Here's how the part is built. I have some questions about the finished solid (model axes, mm). A direction names the side the tool comes from. Round coordinates to 2 decimals unless told otherwise and drop trailing zeros. Loops run counter-clockwise (first coordinate to the right, second up) from the corner with the lowest first, then second, coordinate; pieces in that order, holes last. Notation, with made-up numbers: M -38.75,-12 L 17.25,-12 A25 cw 17.25,9 Z; hole C 65.5,-34 d5. An arc over 180 degrees is marked long. Use a Markdown table: item, result.
from build123d import *

# Parameters (mm, degrees)
SKETCH1_R           = 2.6605
SKETCH1_R_2         = 2.41215
BOSS_EXTRUDE1_DEPTH = 4.5
BOSS_EXTRUDE2_DEPTH = 22.5
SKETCH3_R           = 2.6605
SKETCH3_R_2         = 4.25
BOSS_EXTRUDE3_DEPTH = 4
CUT_EXTRUDE2_DEPTH  = 59.403767002
FILLET1_R           = 4


with BuildPart() as part:
    # Sketch1 → Boss-Extrude1 (new body)
    with BuildSketch(Plane(origin=(0, 0, 0), x_dir=(1, 0, 0), z_dir=(0, 1, 0))):
        with BuildLine():
            Line((-31, -35), (31, -35))
            ThreePointArc((31, -35), (33.828427125, -33.828427125), (35, -31))
            Line((35, -31), (35, 31))
            ThreePointArc((35, 31), (33.828427125, 33.828427125), (31, 35))
            Line((31, 35), (-31, 35))
            ThreePointArc((-31, 35), (-33.828427125, 33.828427125), (-35, 31))
            Line((-35, 31), (-35, -31))
            ThreePointArc((-35, -31), (-33.828427125, -33.828427125), (-31, -35))
        make_face()
        with Locations(Location((25, 22.5, 0), (0, 0, 270))):
            Circle(SKETCH1_R, mode=Mode.SUBTRACT)
        with Locations(Location((25, -22.5, 0), (0, 0, 270))):
            Circle(SKETCH1_R, mode=Mode.SUBTRACT)
        with Locations(Location((-15, -22.5, 0), (0, 0, 270))):
            Circle(SKETCH1_R, mode=Mode.SUBTRACT)
        with Locations(Location((-15, 22.5, 0), (0, 0, 270))):
            Circle(SKETCH1_R, mode=Mode.SUBTRACT)
        with Locations(Location((-12, 0, 0), (0, 0, 270))):
            Circle(SKETCH1_R_2, mode=Mode.SUBTRACT)
        with Locations(Location((-27, 0, 0), (0, 0, 270))):
            Circle(SKETCH1_R_2, mode=Mode.SUBTRACT)
    extrude(amount=BOSS_EXTRUDE1_DEPTH)

    # Sketch2 → Boss-Extrude2 (add)
    with BuildSketch(Plane(origin=(0, 4.5, 0), x_dir=(1, 0, 0), z_dir=(0, 1, 0))):
        with BuildLine():
            Line((-27.289833197, 35), (-31, 35))
            ThreePointArc((-31, 35), (-33.828427125, 33.828427125), (-35, 31))
            Line((-35, 31), (-35, 17))
            Line((-35, 17), (-31.1, 17))
            Line((-31.1, 17), (-31.1, 31))
            ThreePointArc((-31.1, 31), (-31.070710678, 31.070710678), (-31, 31.1))
            Line((-31, 31.1), (-27.289833197, 31.1))
            Line((-27.289833197, 31.1), (-27.289833197, 35))
        make_face()
        with BuildLine():
            Line((-31, -35), (-27.289833197, -35))
            Line((-27.289833197, -35), (-27.289833197, -31.1))
            Line((-27.289833197, -31.1), (-31, -31.1))
            ThreePointArc((-31, -31.1), (-31.070710678, -31.070710678), (-31.1, -31))
            Line((-31.1, -31), (-31.1, -17))
            Line((-31.1, -17), (-35, -17))
            Line((-35, -17), (-35, -31))
            ThreePointArc((-35, -31), (-33.828427125, -33.828427125), (-31, -35))
        make_face()
        with BuildLine():
            Line((17, -35), (31, -35))
            ThreePointArc((31, -35), (33.828427125, -33.828427125), (35, -31))
            Line((35, -31), (35, 31))
            ThreePointArc((35, 31), (33.828427125, 33.828427125), (31, 35))
            Line((31, 35), (17, 35))
            Line((17, 35), (17, 31.1))
            Line((17, 31.1), (31, 31.1))
            ThreePointArc((31, 31.1), (31.070710678, 31.070710678), (31.1, 31))
            Line((31.1, 31), (31.1, -31))
            ThreePointArc((31.1, -31), (31.070710678, -31.070710678), (31, -31.1))
            Line((31, -31.1), (17, -31.1))
            Line((17, -31.1), (17, -35))
        make_face()
    extrude(amount=BOSS_EXTRUDE2_DEPTH)

    # Sketch3 → Boss-Extrude3 (add)
    with BuildSketch(Plane(origin=(0, 27, 0), x_dir=(1, 0, 0), z_dir=(0, 1, 0))):
        with BuildLine():
            Line((-31, 35), (31, 35))
            ThreePointArc((31, 35), (33.828427125, 33.828427125), (35, 31))
            Line((35, 31), (35, -31))
            ThreePointArc((35, -31), (33.828427125, -33.828427125), (31, -35))
            Line((31, -35), (-31, -35))
            ThreePointArc((-31, -35), (-33.828427125, -33.828427125), (-35, -31))
            Line((-35, -31), (-35, 31))
            ThreePointArc((-35, 31), (-33.828427125, 33.828427125), (-31, 35))
        make_face()
        with Locations(Location((-15, 22.5, 0), (0, 0, 270))):
            Circle(SKETCH3_R, mode=Mode.SUBTRACT)
        with Locations(Location((25, 22.5, 0), (0, 0, 270))):
            Circle(SKETCH3_R_2, mode=Mode.SUBTRACT)
        with Locations(Location((25, -22.5, 0), (0, 0, 270))):
            Circle(SKETCH3_R_2, mode=Mode.SUBTRACT)
        with Locations(Location((-15, -22.5, 0), (0, 0, 270))):
            Circle(SKETCH3_R, mode=Mode.SUBTRACT)
        with Locations(Location((-12, 0, 0), (0, 0, 270))):
            Circle(SKETCH3_R_2, mode=Mode.SUBTRACT)
        with Locations(Location((-27, 0, 0), (0, 0, 270))):
            Circle(SKETCH3_R_2, mode=Mode.SUBTRACT)
    extrude(amount=BOSS_EXTRUDE3_DEPTH)

    # Sketch4 → Cut-Extrude2 (cut, through all)
    with BuildSketch(Plane(origin=(0, 0, 0), x_dir=(1, 0, 0), z_dir=(0, 1, 0))):
        with BuildLine():
            Line((-1, -21), (11, -21))
            ThreePointArc((11, -21), (14.535533906, -22.464466094), (16, -26))
            Line((16, -26), (16, -35))
            Line((16, -35), (-6, -35))
            Line((-6, -35), (-6, -26))
            ThreePointArc((-6, -26), (-4.535533906, -22.464466094), (-1, -21))
        make_face()
    extrude(amount=CUT_EXTRUDE2_DEPTH, mode=Mode.SUBTRACT)

    # Fillet1
    fillet1_edges = [part.edges().sort_by_distance(p)[0] for p in [
        (16, 2.25, 35),
        (-6, 2.25, 35),
        (-6, 29, 35),
    ]]
    fillet(fillet1_edges, radius=FILLET1_R)


solid = part.part
1. Imagine slicing it at B-B, the plane x = 25. Write out the boundary of the cut face in (y, z).
Answer sheet:
| item | result |
|---|---|
| outline | M 0,-35 L 31,-35 L 31,-26.75 L 27,-26.75 L 27,-31.1 L 4.5,-31.1 L 4.5,-25.16 L 0,-25.16 Z; M 0,-19.84 L 4.5,-19.84 L 4.5,19.84 L 0,19.84 Z; M 0,25.16 L 4.5,25.16 L 4.5,31.1 L 27,31.1 L 27,26.75 L 31,26.75 L 31,35 L 0,35 Z; M 27,-18.25 L 31,-18.25 L 31,18.25 L 27,18.25 Z |
2. Imagine slicing it at D-D, the plane z = 0. Write out the boundary of the cut face in (x, y), then the cut area to 3 significant figures.
Answer sheet:
| item | result |
|---|---|
| outline | M -35,0 L -29.41,0 L -29.41,4.5 L -35,4.5 Z; M -35,27 L -31.25,27 L -31.25,31 L -35,31 Z; M -24.59,0 L -14.41,0 L -14.41,4.5 L -24.59,4.5 Z; M -22.75,27 L -16.25,27 L -16.25,31 L -22.75,31 Z; M -9.59,0 L 35,0 L 35,31 L -7.75,31 L -7.75,27 L 31.1,27 L 31.1,4.5 L -9.59,4.5 Z |
| area | 571 mm2 |
3. Imagine slicing it at A-A, the plane y = 3.5. Write out the boundary of the cut face in (x, z), then the cut area to 3 significant figures.
Answer sheet:
| item | result |
|---|---|
| outline | M -35,-31 A4 ccw -31,-35 L 31,-35 A4 ccw 35,-31 L 35,31 A4 ccw 31,35 L 20,35 A4 ccw 16,31 L 16,26 A5 cw 11,21 L -1,21 A5 cw -6,26 L -6,31 A4 ccw -10,35 L -31,35 A4 ccw -35,31 Z; hole C -27,0 d4.82; hole C -15,-22.5 d5.32; hole C -15,22.5 d5.32; hole C -12,0 d4.82; hole C 25,-22.5 d5.32; hole C 25,22.5 d5.32 |
| area | 4,460 mm2 |
4. Imagine slicing it at C-C, the plane z = 22.5. State how many separate pieces and enclosed holes the cut face has, then the cut area to 3 significant figures.
Answer sheet:
| item | result |
|---|---|
| separate pieces | 6 |
| enclosed holes | 0 |
| area | 505 mm2 |
5. Which directions (+Z, -Z, +X, -X, +Y, -Y) give clear straight access to the entire face, cutting with the end or side of a thin tool? Please do faces 5 (the face through (-6, 2, 29)), 6 (the face through (27.872, 28.972, -25.632)), 7 (the face through (-27.29, 16, 33)), 8 (the face through (24, 16, -31.1)).
Answer sheet:
| item | result |
|---|---|
| face 5 | +Z, +Y, -Y |
| face 6 | +Y |
| face 7 | +Z, -Z |
| face 8 | none |
6. I need wall thicknesses on probe 1 along Z at (x, y) = (-28, 16.5); probe 2 along Y at (x, z) = (13, -20); probe 3 along X at (y, z) = (29.45, -22.5). Which ranges of each line are inside material? Lowest first, please. Write a range as from..to.
Answer sheet:
| item | result |
|---|---|
| probe 1 | -35..-31.1, 31.1..35 |
| probe 2 | 0..4.5, 27..31 |
| probe 3 | -35..-17.66, -12.34..20.75, 29.25..35 |
7. We'd pull the mould along X, two halves only. Please class faces 1 (the face through (-33.797, 15.283, 33.859)), 2 (the face through (0, 0, 0)), 3 (the face through (33.797, 15.283, -33.859)), 4 (the face through (-29.355, 2.218, -0.523)): +X half, -X half, draft (parallel to the pull), parting line (faces both ways), or undercut.
Answer sheet:
| item | result |
|---|---|
| face 1 | -X half |
| face 2 | draft |
| face 3 | +X half |
| face 4 | undercut |
8. For pin 1 Ø7 at (x, z) = (-15, 22.5) entering from +Y; pin 2 Ø5 at (x, z) = (-27, 0) entering from +Y; pin 3 Ø7 at (y, z) = (20, 13) entering from -X; pin 4 Ø1.9 at (x, y) = (-34, 13) entering from -Z, each with a flat end and sliding along its axis, tell me the tip position at first contact or that it passes through.
Answer sheet:
| item | result |
|---|---|
| pin 1 | y = 31 |
| pin 2 | y = 4.5 |
| pin 3 | x = 31.1 |
| pin 4 | z = -34.43 |
